```python
from build123d import *

# Parameters (mm, degrees)
SKETCH1_R           = 2
SKETCH1_R_2         = 1.25
BOSS_EXTRUDE1_DEPTH = 0.8
BOSS_EXTRUDE2_DEPTH = 1.7
BOSS_EXTRUDE5_START = -5.25
BOSS_EXTRUDE5_DEPTH = 5.25
CUT_EXTRUDE1_DEPTH  = 2.05
CUT_EXTRUDE2_DEPTH  = 5.25
SKETCH4_R           = 3.5
SKETCH4_R_2         = 2
SKETCH4_R_3         = 2.25
SKETCH4_R_4         = 1.25
BOSS_EXTRUDE6_DEPTH = 1.6
CHAMFER1_SIZE       = 1
CUT_EXTRUDE3_START  = -0.5
CUT_EXTRUDE3_DEPTH  = 0.5


with BuildPart() as part:
    # Sketch1 → Boss-Extrude1 (new body)
    with BuildSketch(Plane.XY):
        with BuildLine():
            Line((47.747323671, -3.6), (52.8, -3.6))
            ThreePointArc((52.8, -3.6), (55.133452378, -2.633452378), (56.1, -0.3))
            Line((56.1, -0.3), (56.1, 1.35))
            Line((56.1, 1.35), (54.35, 1.35))
            Line((54.35, 1.35), (54.35, 22.65))
            Line((54.35, 22.65), (56.1, 22.65))
            Line((56.1, 22.65), (56.1, 24.3))
            ThreePointArc((56.1, 24.3), (55.133452378, 26.633452378), (52.8, 27.6))
            Line((52.8, 27.6), (47.745478955, 27.6))
            Line((47.745478955, 27.6), (28.192723723, 27.48950052))
            ThreePointArc((28.192723723, 27.48950052), (26.4684207, 27.34740533), (24.749850743, 27.147582262))
            Line((24.749850743, 27.147582262), (3.864159561, 24.363517328))
            ThreePointArc((3.864159561, 24.363517328), (-1.421825677, 22.090499558), (-3.6, 16.764731413))
            Line((-3.6, 16.764731413), (-3.6, 6.485268587))
            ThreePointArc((-3.6, 6.485268587), (-1.412746343, 1.150273083), (3.890046585, -1.113935993))
            Line((3.890046585, -1.113935993), (25.547001239, -3.33158265))
            ThreePointArc((25.547001239, -3.33158265), (26.875561897, -3.450295565), (28.206747131, -3.534628551))
            Line((28.206747131, -3.534628551), (47.747323671, -3.6))
        make_face()
        with Locations((3.5, 12)):
            Circle(SKETCH1_R, mode=Mode.SUBTRACT)
        with Locations((23.5, 12)):
            Circle(SKETCH1_R, mode=Mode.SUBTRACT)
        with Locations((31.25, 13.75)):
            Circle(SKETCH1_R_2, mode=Mode.SUBTRACT)
        with Locations((31.25, 10.25)):
            Circle(SKETCH1_R_2, mode=Mode.SUBTRACT)
    extrude(amount=BOSS_EXTRUDE1_DEPTH)

    # Sketch1<3> → Boss-Extrude2 (add)
    with BuildSketch(Plane.XY):
        with BuildLine():
            Line((27.968417848, -1.919570033), (27.968417848, 25.870274099))
            ThreePointArc((27.968417848, 25.870274099), (27.217924724, 25.810423929), (26.468417848, 25.739280302))
            Line((26.468417848, 25.739280302), (26.468417848, -1.811733972))
            ThreePointArc((26.468417848, -1.811733972), (27.218012396, -1.871291838), (27.968417848, -1.919570033))
        make_face()
        with BuildLine():
            Line((27.968417848, -2.320209383), (27.968417848, -1.919570033))
            ThreePointArc((27.968417848, -1.919570033), (27.218012396, -1.871291838), (26.468417848, -1.811733972))
            Line((26.468417848, -1.811733972), (26.468417848, -2.213233726))
            ThreePointArc((26.468417848, -2.213233726), (27.21801884, -2.272316396), (27.968417848, -2.320209383))
        make_face()
        with BuildLine():
            ThreePointArc((26.468417848, 25.739280302), (27.217924724, 25.810423929), (27.968417848, 25.870274099))
            Line((27.968417848, 25.870274099), (27.968417848, 26.271306316))
            ThreePointArc((27.968417848, 26.271306316), (27.21793258, 26.21193484), (26.468417848, 26.141360223))
            Line((26.468417848, 26.141360223), (26.468417848, 25.739280302))
        make_face()
    extrude(amount=-BOSS_EXTRUDE2_DEPTH)

    # Sketch1<4> → Boss-Extrude5 (add)
    with BuildSketch(Plane.XY.offset(BOSS_EXTRUDE5_START)):
        with BuildLine():
            Line((28.206747131, -3.534628551), (47.747323671, -3.6))
            Line((47.747323671, -3.6), (52.8, -3.6))
            ThreePointArc((52.8, -3.6), (55.133452378, -2.633452378), (56.1, -0.3))
            Line((56.1, -0.3), (56.1, 1.35))
            Line((56.1, 1.35), (54.35, 1.35))
            Line((54.35, 1.35), (54.35, 22.65))
            Line((54.35, 22.65), (56.1, 22.65))
            Line((56.1, 22.65), (56.1, 24.3))
            ThreePointArc((56.1, 24.3), (55.133452378, 26.633452378), (52.8, 27.6))
            Line((52.8, 27.6), (47.745478955, 27.6))
            Line((47.745478955, 27.6), (28.192723723, 27.48950052))
            ThreePointArc((28.192723723, 27.48950052), (26.4684207, 27.34740533), (24.749850743, 27.147582262))
            Line((24.749850743, 27.147582262), (3.864159561, 24.363517328))
            ThreePointArc((3.864159561, 24.363517328), (-1.421825677, 22.090499558), (-3.6, 16.764731413))
            Line((-3.6, 16.764731413), (-3.6, 6.485268587))
            ThreePointArc((-3.6, 6.485268587), (-1.412746343, 1.150273083), (3.890046585, -1.113935993))
            Line((3.890046585, -1.113935993), (25.547001239, -3.33158265))
            ThreePointArc((25.547001239, -3.33158265), (26.875561897, -3.450295565), (28.206747131, -3.534628551))
        make_face()
        with BuildLine():
            Line((28.235609368, 26.289723719), (47.748869739, 26.4))
            Line((47.748869739, 26.4), (52.8, 26.4))
            ThreePointArc((52.8, 26.4), (54.28492424, 25.78492424), (54.9, 24.3))
            Line((54.9, 24.3), (54.9, 23.85))
            Line((54.9, 23.85), (53.15, 23.85))
            Line((53.15, 23.85), (53.15, 0.15))
            Line((53.15, 0.15), (54.9, 0.15))
            Line((54.9, 0.15), (54.9, -0.3))
            ThreePointArc((54.9, -0.3), (54.28492424, -1.78492424), (52.8, -2.4))
            Line((52.8, -2.4), (47.749330923, -2.4))
            Line((47.749330923, -2.4), (28.239130572, -2.334730172))
            ThreePointArc((28.239130572, -2.334730172), (26.952926693, -2.252708036), (25.669240626, -2.137824914))
            Line((25.669240626, -2.137824914), (3.957730332, 0.085408176))
            ThreePointArc((3.957730332, 0.085408176), (-0.540403389, 1.974754529), (-2.4, 6.485268587))
            Line((-2.4, 6.485268587), (-2.4, 16.764731413))
            ThreePointArc((-2.4, 16.764731413), (-0.542592126, 21.273041161), (3.951517744, 23.164547776))
            Line((3.951517744, 23.164547776), (24.908408379, 25.958103605))
            ThreePointArc((24.908408379, 25.958103605), (26.569258033, 26.151513311), (28.235609368, 26.289723719))
        make_face(mode=Mode.SUBTRACT)
    extrude(amount=BOSS_EXTRUDE5_DEPTH)

    # Sketch2 → Cut-Extrude1 (cut)
    with BuildSketch(Plane(origin=(0, 0, -5.25), x_dir=(-1, 0, 0), z_dir=(0, 0, -1))):
        with BuildLine():
            Line((-27.968417848, 27.474306588), (-27.968417848, 26.271306316))
            ThreePointArc((-27.968417848, 26.271306316), (-26.436023146, 26.138055085), (-24.908408379, 25.958103605))
            Line((-24.908408379, 25.958103605), (-3.951517744, 23.164547776))
            ThreePointArc((-3.951517744, 23.164547776), (0.542592126, 21.273041161), (2.4, 16.764731413))
            Line((2.4, 16.764731413), (2.4, 6.485268587))
            ThreePointArc((2.4, 6.485268587), (0.540403389, 1.974754529), (-3.957730332, 0.085408176))
            Line((-3.957730332, 0.085408176), (-25.669240626, -2.137824914))
            ThreePointArc((-25.669240626, -2.137824914), (-26.817785818, -2.24217071), (-27.968417848, -2.320209383))
            Line((-27.968417848, -2.320209383), (-27.968417848, -3.522067819))
            ThreePointArc((-27.968417848, -3.522067819), (-26.756588582, -3.441074719), (-25.547001239, -3.33158265))
            Line((-25.547001239, -3.33158265), (-3.890046585, -1.113935993))
            ThreePointArc((-3.890046585, -1.113935993), (1.412746343, 1.150273083), (3.6, 6.485268587))
            Line((3.6, 6.485268587), (3.6, 16.764731413))
            ThreePointArc((3.6, 16.764731413), (1.421825677, 22.090499558), (-3.864159561, 24.363517328))
            Line((-3.864159561, 24.363517328), (-24.749850743, 27.147582262))
            ThreePointArc((-24.749850743, 27.147582262), (-26.356573132, 27.336174491), (-27.968417848, 27.474306588))
        make_face()
        with BuildLine():
            ThreePointArc((-24.908408379, 25.958103605), (-26.436023146, 26.138055085), (-27.968417848, 26.271306316))
            Line((-27.968417848, 26.271306316), (-27.968417848, -2.320209383))
            ThreePointArc((-27.968417848, -2.320209383), (-26.817785818, -2.24217071), (-25.669240626, -2.137824914))
            Line((-25.669240626, -2.137824914), (-3.957730332, 0.085408176))
            ThreePointArc((-3.957730332, 0.085408176), (0.540403389, 1.974754529), (2.4, 6.485268587))
            Line((2.4, 6.485268587), (2.4, 16.764731413))
            ThreePointArc((2.4, 16.764731413), (0.542592126, 21.273041161), (-3.951517744, 23.164547776))
            Line((-3.951517744, 23.164547776), (-24.908408379, 25.958103605))
        make_face()
    extrude(amount=-CUT_EXTRUDE1_DEPTH, mode=Mode.SUBTRACT)

    # Sketch3 → Cut-Extrude2 (cut)
    with BuildSketch(Plane(origin=(0, 0, -5.25), x_dir=(-1, 0, 0), z_dir=(0, 0, -1))):
        Polygon((-53.15, 23.85), (-54.9, 23.85), (-54.9, 22.65), (-54.35, 22.65), (-54.35, 1.35), (-54.9, 1.35), (-54.9, 0.15), (-53.15, 0.15), align=None)
    extrude(amount=-CUT_EXTRUDE2_DEPTH, mode=Mode.SUBTRACT)

    # Sketch4 → Boss-Extrude6 (add)
    # profile 1 of 4: a face of its own
    with BuildSketch(Plane.XY.offset(0.8)):
        with Locations((3.5, 12)):
            Circle(SKETCH4_R)
        with Locations((3.5, 12)):
            Circle(SKETCH4_R_2, mode=Mode.SUBTRACT)
    # profile 2 of 4: a face of its own
    with BuildSketch(Plane.XY.offset(0.8)):
        with Locations((23.5, 12)):
            Circle(SKETCH4_R)
        with Locations((23.5, 12)):
            Circle(SKETCH4_R_2, mode=Mode.SUBTRACT)
    # profile 3 of 4: a face of its own
    with BuildSketch(Plane.XY.offset(0.8)):
        with Locations((31.25, 13.75)):
            Circle(SKETCH4_R_3)
        with Locations((31.25, 13.75)):
            Circle(SKETCH4_R_4, mode=Mode.SUBTRACT)
    # profile 4 of 4: a face of its own
    with BuildSketch(Plane.XY.offset(0.8)):
        with Locations((31.25, 10.25)):
            Circle(SKETCH4_R_3)
        with Locations((31.25, 10.25)):
            Circle(SKETCH4_R_4, mode=Mode.SUBTRACT)
    extrude(amount=BOSS_EXTRUDE6_DEPTH)

    # Chamfer1
    chamfer1_edges = [part.edges().sort_by_distance(p)[0] for p in [
        (0, 12, 2.4),
        (20, 12, 2.4),
    ]]
    chamfer(chamfer1_edges, length=CHAMFER1_SIZE)

    # Sketch5 → Cut-Extrude3 (cut)
    with BuildSketch(Plane.XY.offset(2.4).offset(CUT_EXTRUDE3_START)):
        with BuildLine():
            ThreePointArc((32.664213562, 12), (31.25, 16), (29.835786438, 12))
            ThreePointArc((29.835786438, 12), (31.25, 8), (32.664213562, 12))
        make_face()
    extrude(amount=CUT_EXTRUDE3_DEPTH, mode=Mode.SUBTRACT)


solid = part.part
```
The model under review builds one solid part; all positions refer to its coordinate system, in mm. A direction names the side the tool comes from. Coordinates: 2 decimals unless noted, no trailing zeros. Write each loop counter-clockwise with the first axis right and the second up, starting at its lowest first coordinate (ties: lowest second). Pieces come first, ordered by that corner, then holes. Notation, with made-up numbers: (-32, 88) - (12, 88) arc R28 cw to (12, 117) - close; hole circle Ø9 at (1, 72). An arc over 180 degrees is marked (long way). Answer in a Markdown table with one row per item. Add a question column.
Q1. Consider section B-B on x = 23.5. Give the boundary of the cut face in (y, z), then the cut area to 3 significant figures.
Q2. Clearance check with flat-ended pins moving along their axes: pin 1 (3 mm diameter, centred on x = 43.5, z = -3.5, fed in from -Y); pin 2 (0.8 mm diameter, centred on y = 23.5, z = -3, fed in from -X); pin 3 (5 mm diameter, centred on x = 12, y = 19, fed in from -Z). State where each tip first meets the part, or that it passes through.
Q3. For faces 4 (the face through (32.44, 14.13, 0.94)), 5 (the face through (27.968, 12, -1)), list the 3-axis set-ups (+Z, -Z, +X, -X, +Y, -Y) from which the entire face can be reached by the end or side of a thin tool; tool diameter is ignored.
Q4. Draft analysis for pull direction X (two halves, no side actions). For faces 1 (the face through (26.86, -3.45, -1.6)), 2 (the face through (-3, 12, -3.2)), 3 (the face through (50, -2.4, -3)), state which applies: +X half, -X half, draft (parallel to the pull), parting line (faces both ways), or undercut.
Q5. To check wall thickness, follow line 1 along Y through (x, z) = (31.25, 1.3); line 2 along X through (y, z) = (7, -0.25); line 3 along X through (y, z) = (10.25, 1.1). State the ranges of each line that lie inside material, in increasing order. Write a range as from..to.
Q6. Consider section D-D on y = 25. Give the boundary of the cut face in (x, z), then the cut area to 3 significant figures.
Q7. Consider section C-C on x = 52. Give the boundary of the cut face in (y, z), then the cut area to 3 significant figures.
Answers below:
| question | item | result |
|---|---|---|
| 1 | outline | (-3.12, -3.2) - (-1.92, -3.2) - (-1.92, 0) - (10, 0) - (10, 2.4) - (9.5, 2.4) - (8.5, 1.4) - (8.5, 0.8) - (-3.12, 0.8) - close; (14, 0) - (25.77, 0) - (25.77, -3.2) - (26.98, -3.2) - (26.98, 0.8) - (15.5, 0.8) - (15.5, 1.4) - (14.5, 2.4) - (14, 2.4) - close |
| 1 | area | 32.4 mm² |
| 2 | pin 1 | y = -3.59 |
| 2 | pin 2 | x = -0.2 |
| 2 | pin 3 | z = 0 |
| 3 | face 4 | +Z, -Z |
| 3 | face 5 | -Z |
| 4 | face 1 | -X half |
| 4 | face 2 | draft |
| 4 | face 3 | undercut |
| 5 | line 1 | 8..9, 11.5..12.5, 15..16 |
| 5 | line 2 | -3.6..-2.4, 26.47..27.97 |
| 5 | line 3 | 0.47..2.53, 4.47..6.53, 20.47..22.53, 24.47..26.53, 29..30, 32.5..33.5 |
| 6 | outline | (8.64, -3.2) - (17.72, -3.2) - (17.72, 0) - (26.47, 0) - (26.47, -1.7) - (27.97, -1.7) - (27.97, 0) - (54.78, 0) - (54.78, -5.25) - (56.02, -5.25) - (56.02, 0.8) - (8.64, 0.8) - close |
| 6 | area | 76.1 mm² |
| 7 | outline | (-3.6, -5.25) - (-2.4, -5.25) - (-2.4, 0) - (26.4, 0) - (26.4, -5.25) - (27.6, -5.25) - (27.6, 0.8) - (-3.6, 0.8) - close |
| 7 | area | 37.6 mm² |
